CAD build for the part. Positions are in the model's coordinates, mm. A direction names the side the tool comes from. Give positions to 0.01 mm unless a question says otherwise; leave off trailing zeros. Loops run counter-clockwise (first coordinate to the right, second up) from the corner with the lowest first, then second, coordinate; pieces in that order, holes last. Notation, with made-up numbers: M 0,-30.5 L 49,-30.5 A31 cw 49,7.5 Z; hole C -9,76.5 d11. An arc over 180 degrees is marked long. Answer as CSV lines item,"result".
from build123d import *

# Parameters (mm, degrees)
F1_DEPTH = 127
F3_DEPTH = 76.2
F4_SIZE2 = 101.6
F4_SIZE  = 76.2
F5_R     = 5.08
F6_R     = 15.24
F7_DEPTH = 50.8
F8_R     = 12.7
F9_DEPTH = 127


with BuildPart() as f1:
    # F0 (on Front) → F1 (new body)
    with BuildSketch(Plane.XZ):
        Polygon((-38.1, -63.5), (101.6, -63.5), (101.6, 63.5), (0, 63.5), (0, 0), (-38.1, 0), align=None)
        Polygon((-101.6, -63.5), (-38.1, -63.5), (-38.1, 0), (0, 0), (0, 63.5), (-101.6, 63.5), align=None)
    extrude(amount=F1_DEPTH)

    # F2 (on face) → F3 (cut)
    with BuildSketch(Plane.XZ.offset(127)):
        Polygon((-38.1, 0), (-38.1, -63.5), (101.6, -63.5), (101.6, 63.5), (0, 63.5), (0, 0), align=None)
    extrude(amount=-F3_DEPTH, mode=Mode.SUBTRACT)

    # F4
    f4_edges = [f1.edges().sort_by_distance(p)[0] for p in [
        (101.6, -25.4, 63.5),
    ]]
    f4_side = f1.faces().sort_by_distance((-21.771429, -52.614286, 63.5))[0]
    chamfer(f4_edges, length=F4_SIZE, length2=F4_SIZE2, reference=f4_side)

    # F5
    f5_edges = [f1.edges().sort_by_distance(p)[0] for p in [
        (12.7, -50.8, 63.5),
        (25.4, -25.4, 63.5),
        (0, -88.9, 63.5),
        (-50.8, -127, 63.5),
        (0, -127, 31.75),
        (0, -88.9, 0),
        (-19.05, -127, 0),
        (-38.1, -127, -31.75),
        (-38.1, -88.9, -63.5),
        (-69.85, -127, -63.5),
        (-101.6, -127, 0),
        (-101.6, -63.5, 63.5),
        (-38.1, 0, 63.5),
        (-38.1, -50.8, -31.75),
        (-38.1, -88.9, 0),
        (-19.05, -50.8, 0),
        (-101.6, 0, 0),
        (-101.6, -63.5, -63.5),
        (0, 0, -63.5),
        (31.75, -50.8, -63.5),
        (0, -50.8, 31.75),
    ]]
    fillet(f5_edges, radius=F5_R)

    # F6 (on face) → F7 (cut, through all)
    with BuildSketch(Plane.XZ.offset(50.8)):
        with Locations((17.78, -17.78)):
            Circle(F6_R)
    extrude(amount=-F7_DEPTH, mode=Mode.SUBTRACT)

    # F8 (on face) → F9 (cut, through all)
    with BuildSketch(Plane.XY.offset(63.5)):
        with Locations((-77.5449126959, -100.8186563849)):
            Circle(F8_R)
    extrude(amount=-F9_DEPTH, mode=Mode.SUBTRACT)


solid = f1.part
1) Which spindle directions (+Z, -Z, +X, -X, +Y, -Y) get a long thin tool onto all of the face, cutting with end or side? Do faces 4 (the face through (35.232, -49.272, -62.051)), 5 (the face through (0, -89, 32)), 6 (the face through (64.78, -25.04, 10.99)). Say none if no direction does.
Answer below:
face 4,"-Z, +X, -Y"
face 5,"+Z, -Z, +X, -Y"
face 6,"+Z, +X, +Y, -Y"
2) Band-saw the part on C-C on y = -60. Give the cut face in (x, z).
Answer below:
outline,"M -101.6,-58.42 A5.08 ccw -96.52,-63.5 L -43.18,-63.5 A5.08 ccw -38.1,-58.42 L -38.1,-5.08 A5.08 cw -33.02,0 L -5.08,0 A5.08 ccw 0,5.08 L 0,58.42 A5.08 ccw -5.08,63.5 L -96.52,63.5 A5.08 ccw -101.6,58.42 Z"
3) Band-saw the part on A-A on x = 17.78. Give the cut face in (y, z), and give its area (3 significant figures).
Answer below:
outline,"M -50.8,-58.42 A5.08 ccw -45.72,-63.5 L -5.08,-63.5 A5.08 ccw 0,-58.42 L 0,-33.02 L -50.8,-33.02 Z; M -50.8,-2.54 L 0,-2.54 L 0,58.42 A5.08 ccw -5.08,63.5 L -45.72,63.5 A5.08 ccw -50.8,58.42 Z"
area,"4,880 mm^2"
4) Flat gauge pins, fed straight in: pin 1 (14 mm diameter, centred on x = -19.5, y = -98.5, fed in from -Z); pin 2 (6 mm diameter, centred on y = -22.5, z = -28.5, fed in from +X); pin 3 (6 mm diameter, centred on x = 2, z = 3, fed in from -Y). Where does each tip first touch, or does it go through?
Answer below:
pin 1,"stops at z = 0"
pin 2,"stops at x = 96.65"
pin 3,"stops at y = -124.49"
5) Band-saw the part on B-B on z = -17.78. Give the cut face in (x, y), and give its area (3 significant figures).
Answer below:
outline,"M -101.6,-121.92 A5.08 ccw -96.52,-127 L -43.18,-127 A5.08 ccw -38.1,-121.92 L -38.1,-55.88 A5.08 cw -33.02,-50.8 L 2.54,-50.8 L 2.54,0 L -96.52,0 A5.08 ccw -101.6,-5.08 Z; M 33.02,-50.8 L 86.36,-50.8 L 86.36,0 L 33.02,0 Z; hole C -77.54,-100.82 d25.4"
area,"12,300 mm^2"
6) Band-saw the part on D-D on z = 23.5. Give the cut face in (x, y), and give its area (3 significant figures).
Answer below:
outline,"M -101.6,-121.92 A5.08 ccw -96.52,-127 L -5.08,-127 A5.08 ccw 0,-121.92 L 0,-55.88 A5.08 cw 5.08,-50.8 L 55.4,-50.8 L 55.4,0 L -96.52,0 A5.08 ccw -101.6,-5.08 Z; hole C -77.54,-100.82 d25.4"
area,"15,200 mm^2"
7) Mould opens along Y. For faces 1 (the face through (-36.651, -88.438, -1.528)), 2 (the face through (-34.535, -1.449, 61.972)), 3 (the face through (-19.246, -52.249, -1.528)) say: +Y half, -Y half, draft (parallel to the pull), parting line (faces both ways), or undercut.
Answer below:
face 1,"draft"
face 2,"+Y half"
face 3,"-Y half"
8) Drill centre lines: line 1 (Z direction, x = -12, y = -84.5); line 2 (Y direction, x = 65, z = -16.5); line 3 (X direction, y = -90.5, z = -4.5). Where is each one in solid material? Low to high. Write a range as from..to.
Answer below:
line 1,"z = 0..63.5"
line 2,"y = -50.8..0"
line 3,"x = -101.6..-84.95, -70.14..-38.07"
